from build123d import *

# Parameters (mm, degrees)
F1_DEPTH = 11.92
F2_R     = 1.45
F3_DEPTH = 3
F4_R     = 1.45
F5_DEPTH = 3


with BuildPart() as f1:
    # F0 (on Front) → F1 (new body)
    with BuildSketch(Plane.XZ):
        Polygon((2.335372, -0.892208), (1.940361, 1.576388), (-0.395011, 2.468596), (-2.335372, 0.892208), (-1.940361, -1.576388), (0.395011, -2.468596), align=None)
    extrude(amount=F1_DEPTH)

    # F2 (on face) → F3 (join)
    with BuildSketch(Plane(origin=(0, 0, 0), x_dir=(-1, 0, 0), z_dir=(0, 1, 0))):
        Circle(F2_R)
    extrude(amount=F3_DEPTH)

    # F4 (on face) → F5 (cut)
    with BuildSketch(Plane.XZ.offset(11.92)):
        Circle(F4_R)
    extrude(amount=-F5_DEPTH, mode=Mode.SUBTRACT)


solid = f1.part
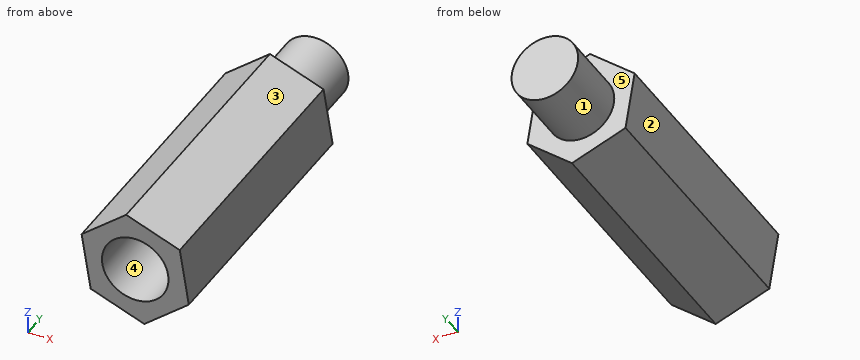
For this review, take the finished solid that the model builds, in its own axes (mm). Face numbers are marked on the shaded views. A direction names the side the tool comes from. Round coordinates to 2 decimals unless told otherwise and drop trailing zeros. Write each loop counter-clockwise with the first axis right and the second up, starting at its lowest first coordinate (ties: lowest second). Pieces come first, ordered by that corner, then holes. Notation, with made-up numbers: M -22,1.25 L 13,1.25 A6 ccw 13,5.25 Z; hole C 69.25,3 d8. An arc over 180 degrees is marked long. Write item = value, one per line. Start each with the question number.
(1) We need section B-B (x = 0). Give the boundary of the cut face in (y, z), then the cut area to 3 significant figures.
(2) The part is to be moulded in two halves that separate along X. For the marked faces 3, 4 and 5, say which applies: +X half, -X half, draft (parallel to the pull), parting line (faces both ways), or undercut.
(3) For line 1 along Y through (x, z) = (0.55, -2.3); line 2 along Y through (x, z) = (1.1, -0.7); line 3 along Z through (x, y) = (0, -10.85), list the stretches that pass through material, from the lowest coordinate up.
(4) We need section C-C (z = 0). Give the boundary of the cut face in (x, y).
(5) We need section A-A (y = -7.5). Give the boundary of the cut face in (x, z), then the cut area to 3 significant figures.
(6) Clearance check with a flat-ended pin moving along its axis: pin 1 Ø2.5 at (x, z) = (0, 0) entering from -Y. State where the tip first meets the part, or that it passes through.
(7) We need section D-D (y = 2). Give the boundary of the cut face in (x, z), then the cut area to 3 significant figures.
(8) For the marked faces 1 and 2, list the 3-axis set-ups (+Z, -Z, +X, -X, +Y, -Y) from which the entire face can be reached by the end or side of a thin tool; tool diameter is ignored.
Results found:
q1.outline = M -11.92,-2.32 L 0,-2.32 L 0,-1.45 L 3,-1.45 L 3,1.45 L 0,1.45 L 0,2.32 L -11.92,2.32 L -11.92,1.45 L -8.92,1.45 L -8.92,-1.45 L -11.92,-1.45 Z
q1.area = 55.3 mm²
q2.face_3 = +X half
q2.face_4 = undercut
q2.face_5 = draft
q3.line_1 = -11.92 to 0
q3.line_2 = -8.92 to 3
q3.line_3 = -2.32 to -1.45, 1.45 to 2.32
q4.outline = M -2.19,-11.92 L -1.45,-11.92 L -1.45,-8.92 L 1.45,-8.92 L 1.45,-11.92 L 2.19,-11.92 L 2.19,0 L 1.45,0 L 1.45,3 L -1.45,3 L -1.45,0 L -2.19,0 Z
q5.outline = M -2.34,0.89 L -1.94,-1.58 L 0.4,-2.47 L 2.34,-0.89 L 1.94,1.58 L -0.4,2.47 Z
q5.area = 16.2 mm²
q6.pin_1 = -8.92
q7.outline = C 0,0 d2.9
q7.area = 6.61 mm²
q8.face_1 = +Y
q8.face_2 = -Z, -X, +Y, -Y
